Check sheet for the modelled part. Datum: model origin and axes. Units: mm. A direction names the side the tool comes from. Round coordinates to 2 decimals unless told otherwise and drop trailing zeros. Write each loop counter-clockwise with the first axis right and the second up, starting at its lowest first coordinate (ties: lowest second). Pieces come first, ordered by that corner, then holes. Notation, with made-up numbers: (-40, 19.5) -> (-10, 19.5) arc R17 ccw to (-10, 47.5) -> close; hole circle Ø11 at (-14.5, 68.25). An arc over 180 degrees is marked (long way). One line per item, written item: value.
from build123d import *

# Parameters (mm, degrees)
F1_DEPTH = 5
F2_R     = 1.5
F3_DEPTH = 6
F4_R     = 1.25
F5_DEPTH = 4


with BuildPart() as f1:
    # F0 (on Top) → F1 (new body)
    with BuildSketch(Plane.XY):
        Polygon((1.587713, 2.75), (-1.587713, 2.75), (-3.175426, 0), (-1.587713, -2.75), (1.587713, -2.75), (3.175426, 0), align=None)
    extrude(amount=F1_DEPTH)

    # F2 (on face) → F3 (join)
    with BuildSketch(Plane.XY.offset(5)):
        Circle(F2_R)
    extrude(amount=F3_DEPTH)

    # F4 (on face) → F5 (cut)
    with BuildSketch(Plane(origin=(0, 0, 0), x_dir=(1, 0, 0), z_dir=(0, 0, -1))):
        Circle(F4_R)
    extrude(amount=-F5_DEPTH, mode=Mode.SUBTRACT)


solid = f1.part
Item 1: Sectioned sample at D-D on z = 6.75. Enter the section's corners in (x, y), and give its area (3 significant figures).
Answer:
outline: circle Ø3 at (0, 0)
area: 7.07 mm^2
Item 2: Tool access check on faces 4 (the flat face through (0, 0, 11)), 5 (the cylindrical face through (-0.27, 1.22, 1.97)). Record the directions out of +Z, -Z, +X, -X, +Y, -Y that give a thin tool (end or side, any length) a straight path to the whole face; none if there is none.
Answer:
face 4: +Z, +X, -X, +Y, -Y
face 5: -Z
Item 3: Thickness scan on line 1 (Y direction, x = 0, z = 0.9); line 2 (X direction, y = 0.1, z = 9); line 3 (Z direction, x = -0.75, y = -0.2). Record the ranges inside material, lowest first.
Answer:
line 1: y = -2.75 to -1.25, 1.25 to 2.75
line 2: x = -1.5 to 1.5
line 3: z = 4 to 11
Item 4: Sectioned sample at A-A on z = 2. Enter the section's corners in (x, y).
Answer:
outline: (-3.18, 0) -> (-1.59, -2.75) -> (1.59, -2.75) -> (3.18, 0) -> (1.59, 2.75) -> (-1.59, 2.75) -> close; hole circle Ø2.5 at (0, 0)
Item 5: Sectioned sample at B-B on x = 0. Enter the section's corners in (y, z), and give its area (3 significant figures).
Answer:
outline: (-2.75, 0) -> (-1.25, 0) -> (-1.25, 4) -> (1.25, 4) -> (1.25, 0) -> (2.75, 0) -> (2.75, 5) -> (1.5, 5) -> (1.5, 11) -> (-1.5, 11) -> (-1.5, 5) -> (-2.75, 5) -> close
area: 35.5 mm^2
Item 6: Depth check by flat-ended pin: P1, Ø3, axis at x = 0.5, z = 9, coming from the -Y side; P2, Ø1.5, axis at x = 0, y = 0, coming from the -Z side; P3, Ø2, axis at x = 0, y = -0.5, coming from the -Z side. Enter the tip coordinate at first touch or a pass-through.
Answer:
P1: stops at y = -1.5
P2: stops at z = 4
P3: stops at z = 0
Item 7: Sectioned sample at C-C on y = 0.55. Enter the section's corners in (x, z), and give its area (3 significant figures).
Answer:
outline: (-2.86, 0) -> (-1.12, 0) -> (-1.12, 4) -> (1.12, 4) -> (1.12, 0) -> (2.86, 0) -> (2.86, 5) -> (1.4, 5) -> (1.4, 11) -> (-1.4, 11) -> (-1.4, 5) -> (-2.86, 5) -> close
area: 36.3 mm^2
Item 8: Mould release check, pull along X, two halves, no side actions. Record for faces 1 (the cylindrical face through (-1.5, 0.07, 7.96)), 2 (the flat face through (1.4, 1.3, 5)), 3 (the flat face through (0, 0, 4)): pulls with the +X half, pulls with the -X half, needs draft (parallel to the pull), parting line crosses it, or undercut.
Answer:
face 1: parting line crosses it
face 2: needs draft
face 3: undercut
